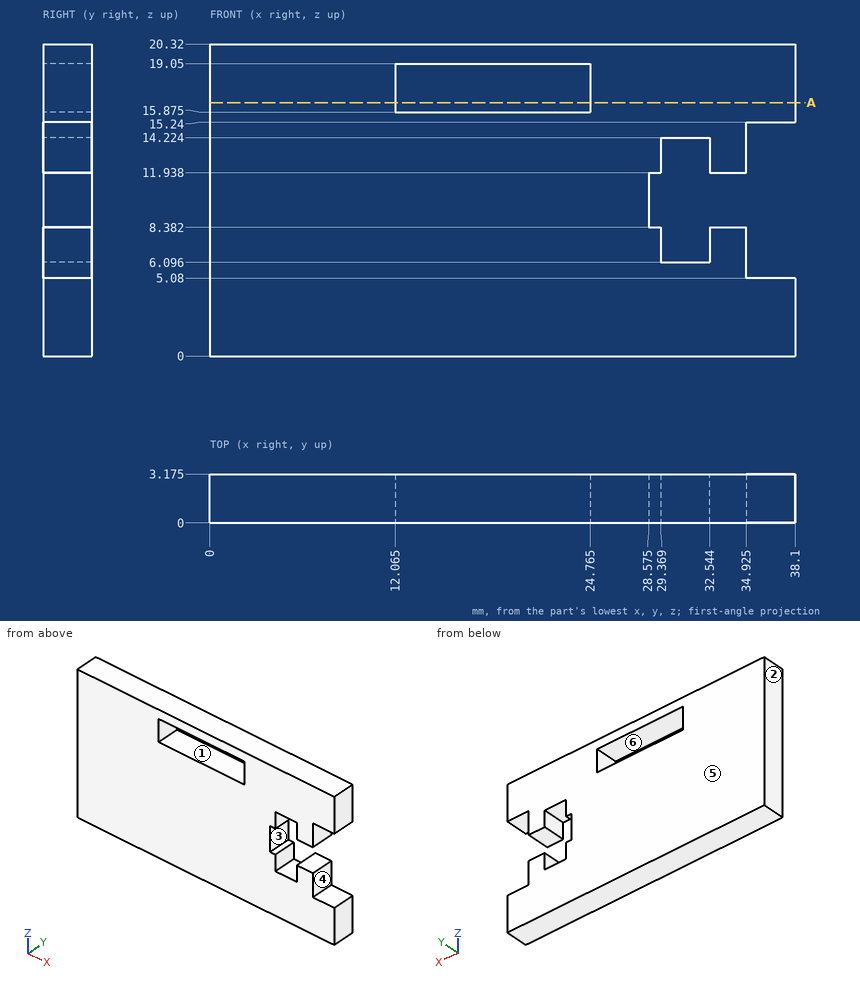
Answer from the drawing. Dimensions are ordinates in mm from the lowest x, y and z of the part. A direction names the side the tool comes from. Give positions to 0.01 mm unless a question says otherwise; leave off trailing zeros. Order: outer loops, then holes, each group sorted by start corner. A loop starts at its lowest first (then second) coordinate and runs counter-clockwise, first axis right, second up. Notation, with made-up numbers: (50, 79.25) - (99, 79.25) arc R10 cw to (99, 97.25) - close; hole circle Ø5 at (7, 35.5). An arc over 180 degrees is marked (long way). One line per item, written item: value. Start each with the question number.
1. Consider line 1 (X direction, y = 0.95, z = 8) (1 decimal); line 2 (Z direction, x = 32.5, y = 3); line 3 (X direction, y = 2.9, z = 14.5) (1 decimal). Determine where each line is inside the solid, lowest interval first.
2. This flat-tipped pin is pushed along its axis until it touches: pin 1 Ø1 at (y, z) = (2.5, 6) entering from +X (3 decimals). Where does it stop, or does it pass through?
3. For a pull along X with two mould halves and no side action, classify the marked faces 4, 5 and 6 as released by +X, released by -X, zero draft, split by the parting line, or undercut.
4. Section A-A, the plane z = 16.5 is taken. Write down the section's boundary in (x, y) (1 decimal).
5. Which of the six approach directions +Z, -Z, +X, -X, +Y, -Y give full straight-line access (tool end or side, diameter ignored) to the marked faces 1, 2 and 3?
Filled sheet:
1. line 1: 0 to 29.4, 32.5 to 34.9
1. line 2: 0 to 6.1, 14.22 to 20.32
1. line 3: 0 to 34.9
2. pin 1: x = 34.925
3. face 4: released by +X
3. face 5: zero draft
3. face 6: undercut
4. outline: (0, 0) - (12.1, 0) - (12.1, 3.2) - (0, 3.2) - close; (24.8, 0) - (38.1, 0) - (38.1, 3.2) - (24.8, 3.2) - close
5. face 1: +Y, -Y
5. face 2: +Z, -Z, -X, +Y, -Y
5. face 3: +X, +Y, -Y
